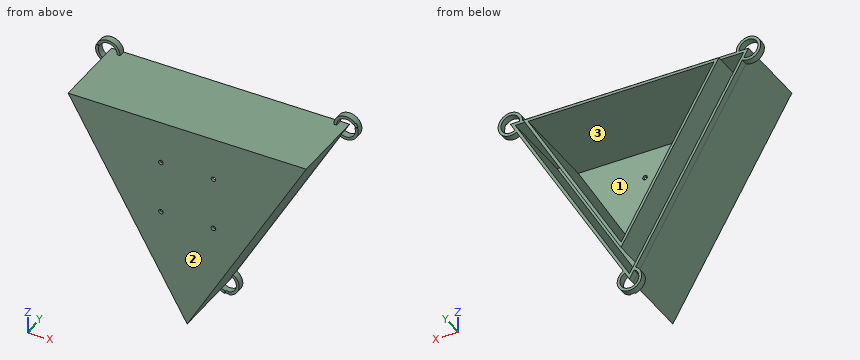
```python
from build123d import *

# Parameters (mm, degrees)
BOSS_EXTRUDE1_DEPTH          = 3.5
CUT_EXTRUDE1_DEPTH           = 0.5
CUT_EXTRUDE2_DEPTH           = 0.5
CUT_EXTRUDE3_DEPTH           = 0.5
BOSS_EXTRUDE2_DEPTH          = 38
CUT_EXTRUDE4_DEPTH           = 40
BOSS_EXTRUDE3_DEPTH          = 48
CUT_EXTRUDE5_DEPTH           = 48
F_2_45_2_45_DIAMETER_HOLE1_D = 2.45


with BuildPart() as part:
    # Sketch1 → Boss-Extrude1 (new body)
    with BuildSketch(Plane.XZ.offset(-38)):
        with BuildLine():
            Line((3.25, -67.370834875), (59.969854476, 30.870834875))
            ThreePointArc((59.969854476, 30.870834875), (68.849019601, 39.75), (56.719854476, 36.5))
            Line((56.719854476, 36.5), (-56.719854476, 36.5))
            ThreePointArc((-56.719854476, 36.5), (-68.849019601, 39.75), (-59.969854476, 30.870834875))
            Line((-59.969854476, 30.870834875), (-3.25, -67.370834875))
            ThreePointArc((-3.25, -67.370834875), (0, -79.5), (3.25, -67.370834875))
        make_face()
        with BuildLine():
            Line((-2.5, -68.669872981), (0, -73))
            Line((0, -73), (2.5, -68.669872981))
            ThreePointArc((2.5, -68.669872981), (0, -78), (-2.5, -68.669872981))
        make_face(mode=Mode.SUBTRACT)
        with BuildLine():
            Line((-58.219854476, 36.5), (-63.219854476, 36.5))
            Line((-63.219854476, 36.5), (-60.719854476, 32.169872981))
            ThreePointArc((-60.719854476, 32.169872981), (-67.549981495, 39), (-58.219854476, 36.5))
        make_face(mode=Mode.SUBTRACT)
        with BuildLine():
            Line((60.719854476, 32.169872981), (63.219854476, 36.5))
            Line((63.219854476, 36.5), (58.219854476, 36.5))
            ThreePointArc((58.219854476, 36.5), (67.549981495, 39), (60.719854476, 32.169872981))
        make_face(mode=Mode.SUBTRACT)
    extrude(amount=-BOSS_EXTRUDE1_DEPTH)

    # Sketch2 → Cut-Extrude1 (cut)
    with BuildSketch(Plane.XZ.offset(-38)):
        with BuildLine():
            Line((1.128713155, -79.401250395), (0.868240888, -77.924038765))
            ThreePointArc((0.868240888, -77.924038765), (0, -78), (-0.868240888, -77.924038765))
            Line((-0.868240888, -77.924038765), (-1.128713155, -79.401250395))
            ThreePointArc((-1.128713155, -79.401250395), (0, -79.5), (1.128713155, -79.401250395))
        make_face()
    extrude(amount=-CUT_EXTRUDE1_DEPTH, mode=Mode.SUBTRACT)

    # Sketch3 → Cut-Extrude2 (cut)
    with BuildSketch(Plane.XZ.offset(-38)):
        with BuildLine():
            Line((-69.327856511, 38.723130932), (-67.91831758, 38.210100717))
            ThreePointArc((-67.91831758, 38.210100717), (-67.549981495, 39), (-67.050076692, 39.713938048))
            Line((-67.050076692, 39.713938048), (-68.199143357, 40.678119463))
            ThreePointArc((-68.199143357, 40.678119463), (-68.849019601, 39.75), (-69.327856511, 38.723130932))
        make_face()
    extrude(amount=-CUT_EXTRUDE2_DEPTH, mode=Mode.SUBTRACT)

    # Sketch4 → Cut-Extrude3 (cut)
    with BuildSketch(Plane.XZ.offset(-38)):
        with BuildLine():
            Line((67.91831758, 38.210100717), (69.327856511, 38.723130932))
            ThreePointArc((69.327856511, 38.723130932), (68.849019601, 39.75), (68.199143357, 40.678119463))
            Line((68.199143357, 40.678119463), (67.050076692, 39.713938048))
            ThreePointArc((67.050076692, 39.713938048), (67.549981495, 39), (67.91831758, 38.210100717))
        make_face()
    extrude(amount=-CUT_EXTRUDE3_DEPTH, mode=Mode.SUBTRACT)

    # Sketch5 → Boss-Extrude2 (add)
    with BuildSketch(Plane.XZ.offset(-38)):
        Polygon((0, -73), (-63.219854476, 36.5), (63.219854476, 36.5), align=None)
    extrude(amount=BOSS_EXTRUDE2_DEPTH)

    # Sketch6 → Cut-Extrude4 (cut)
    with BuildSketch(Plane(origin=(0, 41.5, 0), x_dir=(-1, 0, 0), z_dir=(0, 1, 0))):
        Polygon((0, -70), (60.621778265, 35), (-60.621778265, 35), align=None)
    extrude(amount=-CUT_EXTRUDE4_DEPTH, mode=Mode.SUBTRACT)

    # Sketch7 → Boss-Extrude3 (add)
    with BuildSketch(Plane(origin=(0, 1.5, 0), x_dir=(-1, 0, 0), z_dir=(0, 1, 0))):
        Polygon((0, -60), (-51.961524227, 30), (51.961524227, 30), align=None)
    extrude(amount=BOSS_EXTRUDE3_DEPTH)

    # Sketch8 → Cut-Extrude5 (cut)
    with BuildSketch(Plane(origin=(0, 49.5, 0), x_dir=(-1, 0, 0), z_dir=(0, 1, 0))):
        Polygon((49.363448016, 28.5), (-49.363448016, 28.5), (0, -57), align=None)
    extrude(amount=-CUT_EXTRUDE5_DEPTH, mode=Mode.SUBTRACT)

    # Ø2.45 (2.45) Diameter Hole1 (through all)
    with Locations(Plane(origin=(0, 1.5, 0), x_dir=(1, 0, 0), z_dir=(0, 1, 0))):
        with Locations((-13.95, 13.95), (13.95, -13.95), (-13.95, -13.95), (13.95, 13.95)):
            Hole(F_2_45_2_45_DIAMETER_HOLE1_D / 2)


solid = part.part
```
CAD build for the part. Positions are in the model's coordinates, mm. Face numbers are marked on the shaded views. Coordinates: 2 decimals unless noted, no trailing zeros. Write each loop counter-clockwise with the first axis right and the second up, starting at its lowest first coordinate (ties: lowest second). Pieces come first, ordered by that corner, then holes.
(1) Two-plate mould, pull along Z, no slides. Class the marked faces 1, 2 and 3: +Z half, -Z half, draft (parallel to the pull), parting line (faces both ways), or undercut.
(2) Cut at D-D, the plane x = 11. List the corners of the cut face in (y, z).
(3) Cut at A-A, the plane y = 23.5. List the corners of the cut face in (x, z), and give its area (3 significant figures).
(4) Cut at C-C, the plane z = -28.5. List the corners of the cut face in (x, y), and give its area (3 significant figures).
(5) Cut at B-B, the plane y = 44. List the corners of the cut face in (x, z), and give its area (3 significant figures).
(6) Flat gauge pins, fed straight in: pin 1 (10 mm diameter, centred on x = -49.5, y = 33.5, fed in from +Z); pin 2 (12 mm diameter, centred on x = -37.5, y = 15, fed in from -Z); pin 3 (10 mm diameter, centred on x = -10, y = 40, fed in from -Z); pin 4 (4.5 mm diameter, centred on x = -62.5, z = 35, fed in from -Y). Where does each tip first touch, or does it go through?
(7) Drill centre lines: probe 1 along Z at (x, y) = (0, 39.8); probe 2 along Z at (x, y) = (-16.5, 18); probe 3 along Z at (x, y) = (-13, 1). Where is each one in solid material? Low to high.
Geometry says:
1. face 1: undercut
1. face 2: draft
1. face 3: undercut
2. outline: (0, -53.95) - (41.5, -53.95) - (41.5, -50.95) - (1.5, -50.95) - (1.5, -40.95) - (49.5, -40.95) - (49.5, -37.95) - (1.5, -37.95) - (1.5, 28.5) - (49.5, 28.5) - (49.5, 30) - (1.5, 30) - (1.5, 35) - (41.5, 35) - (41.5, 36.5) - (0, 36.5) - close
3. outline: (-63.22, 36.5) - (0, -73) - (63.22, 36.5) - close; (-51.96, 30) - (0, -60) - (51.96, 30) - close; hole (-60.62, 35) - (0, -70) - (60.62, 35) - close; hole (-49.36, 28.5) - (0, -57) - (49.36, 28.5) - close
3. area: 1,010 mm2
4. outline: (-25.69, 0) - (25.69, 0) - (25.69, 41.5) - (23.96, 41.5) - (23.96, 1.5) - (18.19, 1.5) - (18.19, 49.5) - (16.45, 49.5) - (16.45, 1.5) - (-16.45, 1.5) - (-16.45, 49.5) - (-18.19, 49.5) - (-18.19, 1.5) - (-23.96, 1.5) - (-23.96, 41.5) - (-25.69, 41.5) - close
4. area: 382 mm2
5. outline: (-51.96, 30) - (0, -60) - (51.96, 30) - close; hole (-49.36, 28.5) - (0, -57) - (49.36, 28.5) - close
5. area: 456 mm2
6. pin 1: stops at z = 36.5
6. pin 2: stops at z = -18.44
6. pin 3: stops at z = -77.15
6. pin 4: stops at y = 0
7. probe 1: z = -79.5 to -78, -73 to -70, -60 to -57, 28.5 to 30, 35 to 36.5
7. probe 2: z = -44.42 to -41.42, -31.42 to -28.42, 28.5 to 30, 35 to 36.5
7. probe 3: z = -50.48 to -14.72, -13.18 to 13.18, 14.72 to 36.5
